```python
from build123d import *

# Parameters (mm, degrees)
SKETCH_1_W                   = 18.55
SKETCH_1_H                   = 30
EXTRUDE_1_DEPTH              = 1.5
HOLE_WIZARD_M4_1_D           = 4.5
HOLE_WIZARD_M4_1_DEPTH       = 3
HOLE_WIZARD_M4_1_CSINK_D     = 4.55
HOLE_WIZARD_M4_1_CSINK_ANGLE = 92


with BuildPart() as part:
    # 스케치1 → 보스-돌출1 (new body, symmetric)
    with BuildSketch(Plane.XY):
        Rectangle(SKETCH_1_W, SKETCH_1_H)
    extrude(amount=EXTRUDE_1_DEPTH, both=True)

    # M4 여유 구멍1
    with Locations(Plane.XY.offset(1.5)):
        with Locations((-4, -5.005), (4, 5.005), (-4, 5.005), (4, -5.005)):
            CounterSinkHole(HOLE_WIZARD_M4_1_D / 2, HOLE_WIZARD_M4_1_CSINK_D / 2, depth=HOLE_WIZARD_M4_1_DEPTH, counter_sink_angle=HOLE_WIZARD_M4_1_CSINK_ANGLE)


solid = part.part
```
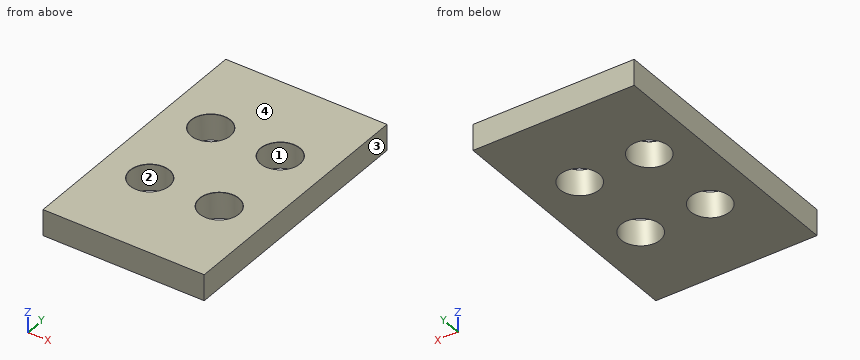
The listing builds one solid part. Answer for the finished solid, in the listing's coordinates (mm). Face numbers are marked on the shaded views. Give positions to 0.01 mm unless a question says otherwise; leave off trailing zeros. Order: outer loops, then holes, each group sorted by start corner. A loop starts at its lowest first (then second) coordinate and runs counter-clockwise, first axis right, second up. Notation, with made-up numbers: (67, -11.5) - (97, -11.5) arc R19 cw to (97, 3.5) - close; hole circle Ø1 at (-18, -37.5). An arc over 180 degrees is marked (long way). Use one line per item in the form item = value. Start each with the question number.
(1) A cutting plane is placed at A-A, the plane x = 4. Write down the section's boundary in (y, z) (3 decimals), then the cut area to 3 significant figures.
(2) The mould has two halves that part along X. Classify the marked faces 1, 2, 3 and 4: released by +X, released by -X, zero draft, split by the parting line, or undercut.
(3) A cutting plane is placed at C-C, the plane x = -5.75. State how many separate pieces and enclosed holes the cut face has, then the cut area to 3 significant figures.
(4) Flat-ended cylindrical pins translate along their axes: pin 1 Ø6 at (x, y) = (-3.5, -4) entering from -Z; pin 2 Ø4 at (x, y) = (4, -5.005) entering from +Z. Find the tip coordinate at first contact, or state that the pin passes through.
(5) A cutting plane is placed at B-B, the plane z = -0.8. Write down the section's boundary in (x, y) (3 decimals), then the cut area to 3 significant figures.
(6) Consider line 1 (Y direction, x = -4, z = 0.8) (3 decimals); line 2 (Y direction, x = 4.25, z = 0.6); line 3 (X direction, y = 3, z = 0.1) (3 decimals). Determine where each line is inside the solid, lowest interval first. Write a range as from..to.
Ans:
q1.outline = (-15, -1.5) - (-7.255, -1.5) - (-7.255, 1.476) - (-7.28, 1.5) - (-15, 1.5) - close; (-2.755, -1.5) - (2.755, -1.5) - (2.755, 1.476) - (2.73, 1.5) - (-2.73, 1.5) - (-2.755, 1.476) - close; (7.255, -1.5) - (15, -1.5) - (15, 1.5) - (7.28, 1.5) - (7.255, 1.476) - close
q1.area = 63.0 mm^2
q2.face_1 = undercut
q2.face_2 = undercut
q2.face_3 = released by +X
q2.face_4 = zero draft
q3.separate_pieces = 3
q3.enclosed_holes = 0
q3.area = 73.0 mm^2
q4.pin_1 = -1.5
q4.pin_2 = through
q5.outline = (-9.275, -15) - (9.275, -15) - (9.275, 15) - (-9.275, 15) - close; hole circle Ø4.5 at (-4, -5.005); hole circle Ø4.5 at (-4, 5.005); hole circle Ø4.5 at (4, -5.005); hole circle Ø4.5 at (4, 5.005)
q5.area = 493 mm^2
q6.line_1 = -15..-7.255, -2.755..2.755, 7.255..15
q6.line_2 = -15..-7.24, -2.77..2.77, 7.24..15
q6.line_3 = -9.275..-5.021, -2.979..2.979, 5.021..9.275
